Autodesk Inventor part; units mm, degrees
ref_plane "Work Plane1" through (9, 0, 0) normal (1, 0, 0) x (0, 0, -1)
ref_plane "YZ Plane" through (0, 0, 0) normal (1, 0, 0) x (0, 1, 0)
ref_plane "XZ Plane" through (0, 0, 0) normal (0, 1, 0) x (-1, 0, 0)
sketch "Sketch1" plane through (0, 0, 0) normal (1, 0, 0) x (0, 1, 0)
  circle A0 centre (0, 0) radius 1.4
  line L0 (0.5, 1.30767) -> (0.5, -1.30767)
  dimension "d1" = 2.8
  dimension "d2" = 0.5
extrude "Extrusion1" add sketch "Sketch1" along normal blind 8 contours L0 A0 picked at (-0.62029, 0.295862)
sketch "Sketch2" plane through (0, 0, 0) normal (-1, 0, 0) x (0, 0, 1)
  circle A0 centre (0, 0) radius 8.75
  arc A1 (-1.30767, 0.5) -> (1.30767, 0.5) centre (0, 0) ccw
  dimension "d5" = 17.5
extrude "Extrusion2" add sketch "Sketch2" along normal blind 8
sketch "Sketch3" plane through (0, 0, 0) normal (1, 0, 0) x (0, 1, 0)
  circle A0 centre (0, 0) radius 4.25
  line L0 (4, 1.75) -> (8.573214, 1.75)
  line L1 (4, -1.75) -> (8.573214, -1.75)
  line L2 (-10.5, 0) -> (10.5, 0)
  circle A1 centre (0, 0) radius 8.75
  line L3 (0.5, -1.30767) -> (0.5, 1.30767)
  arc A2 (0.5, 1.30767) -> (0.5, -1.30767) centre (0, 0) ccw
  arc A3 (3.820225, 1.86236) -> (4, 1.75) centre (4, 1.95) ccw
  arc A4 (4, -1.75) -> (3.820225, -1.86236) centre (4, -1.95) ccw
  line L4 (-3.515544, 2.589102) -> (-5.802152, 6.549621)
  line L5 (-0.484456, 4.339102) -> (-2.771063, 8.299621)
  arc A5 (-0.484456, 4.339102) -> (-0.297262, 4.239591) centre (-0.31125, 4.439102) ccw
  arc A6 (-3.522963, 2.377232) -> (-3.515544, 2.589102) centre (-3.68875, 2.489102) ccw
  line L6 (-0.484456, -4.339102) -> (-2.771063, -8.299621)
  line L7 (-3.515544, -2.589102) -> (-5.802152, -6.549621)
  arc A7 (-3.515544, -2.589102) -> (-3.522963, -2.377232) centre (-3.68875, -2.489102) ccw
  arc A8 (-0.297262, -4.239591) -> (-0.484456, -4.339102) centre (-0.31125, -4.439102) ccw
  arc A9 (0.5, 1.30767) -> (0.5, -1.30767) centre (0, 0) ccw
  circle A10 centre (0, 0) radius 5
  line L8 (4, 1.75) -> (3.872983, 1.75)
  line L9 (4, -1.75) -> (3.840573, -1.75)
  line L10 (-0.484456, -4.339102) -> (-0.420947, -4.229102)
  line L11 (-3.515544, -2.589102) -> (-3.452036, -2.479102)
  line L12 (-3.515544, 2.589102) -> (-3.452036, 2.479102)
  line L13 (-0.484456, 4.339102) -> (-0.420947, 4.229102)
  point P0 (-3.522963, -2.377232)
  point P1 (-4.25, 0)
  point P2 (-8.75, 0)
  point P3 (-5.802152, -6.549621)
  point P4 (-0.297262, -4.239591)
  point P5 (-2.771063, -8.299621)
  point P6 (8.573214, -1.75)
  point P7 (-0.297262, 4.239591)
  point P8 (-3.522963, 2.377232)
  point P9 (-5.802152, 6.549621)
  point P10 (3.872983, -1.75)
  dimension "d8" = 8.5
  dimension "d9" = 3.5
  dimension "d10" = 4
  dimension "d14" = 360
  dimension "d22" = 10
extrude "Extrusion3" add sketch "Sketch3" along normal blind 8 contours A0 A3 L8 | L9 A4 A0 | A0 A5 L5 A10 L0 A3 | A4 L1 A10 L6 A8 A0 | A10 L5 A1 L0 | L1 A1 L6 A10 | A0 L13 A5 | A8 L10 A0 | L2 A10 L4 A6 A0 | A0 A7 L7 A10 L2 | A10 L2 A1 L4 | L7 A1 L2 A10 | A6 L12 A0 | A0 L11 A7
sketch "Sketch4" plane through (-8, 0, 0) normal (-1, 0, 0) x (0, 0, 1)
  circle A0 centre (0, 0) radius 6.65
  dimension "d19" = 13.3
extrude "Extrusion4" cut sketch "Sketch4" against normal blind 5.5
fillet "Fillet1" radius 3 6 edges at (4, 3.873, 1.75) (4, -0.4209, 4.2291) (4, 3.873, -1.75) (4, -0.4209, -4.2291) (4, -3.452, -2.4791) (4, -3.452, 2.4791)
sketch "Sketch5" plane through (-2.5, 0, 0) normal (-1, 0, 0) x (0, 0, 1)
  circle A0 centre (0, 0) radius 2.5
  dimension "d24" = 5
extrude "Extrusion5" [suppressed]
sketch "Sketch6" plane through (-22, 0, 0) normal (-1, 0, 0) x (0, 0, 1)
  arc A0 (-1.2, 0.5) -> (1.2, 0.5) centre (0, 0) ccw
  circle A1 centre (0, 0) radius 2.5
ref_plane "Work Plane1" through (9, 0, 0) normal (1, 0, 0) x (0, 0, -1)
sketch "Sketch7" plane through (9, 0, 0) normal (1, 0, 0) x (0, 0, -1)
  arc A0 (-1.30767, 0.5) -> (1.30767, 0.5) centre (0, 0) ccw
  line L0 (1.30767, 0.5) -> (-1.30767, 0.5)
  circle A1 centre (0, 0) radius 1.6
  line L1 (-1.438749, 0.7) -> (1.438749, 0.7)
  dimension "d28" = 3.2
  dimension "d30" = 0.5
  dimension "d31" = 0.7
sketch "Sketch8" plane through (8, 0, 0) normal (1, 0, 0) x (0, 0, -1)
  arc A0 (-1.30767, 0.5) -> (1.30767, 0.5) centre (0, 0) ccw
  line L0 (1.30767, 0.5) -> (-1.30767, 0.5)
sketch "Sketch7 outline for Loft1" plane through (9, 0, 0) normal (1, 0, 0) x (0, 0, -1)
  line L0 (1.438749, 0.7) -> (-1.438749, 0.7)
  arc A0 (-1.438749, 0.7) -> (1.438749, 0.7) centre (0, 0) ccw
loft "Loft1" add profiles "Sketch7 outline for Loft1" section 1 edges at (8, -1.4, 0) (8, 0.5, 0)
sketch "Sketch9" plane through (-2.5, 0, 0) normal (-1, 0, 0) x (0, 0, 1)
  circle A0 centre (0, 0) radius 3.15
  dimension "d36" = 6.3
extrude "Extrusion6" cut sketch "Sketch9" against normal blind 0.4
properties part number "front wheel mount"
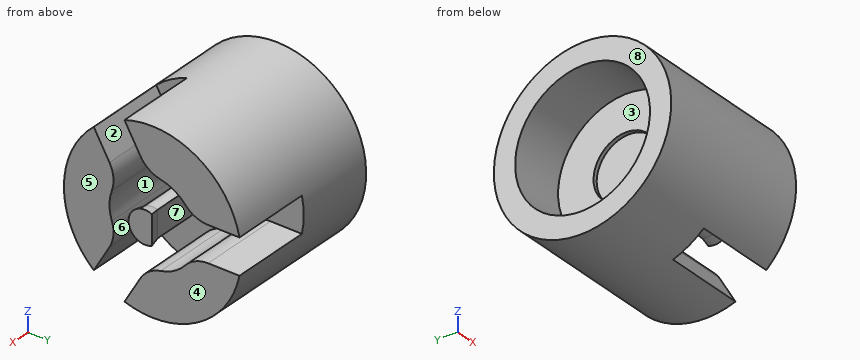
Verification items for the finished model (mm, model axes). Face numbers are marked on the shaded views. A direction names the side the tool comes from. Coordinates: 2 decimals unless noted, no trailing zeros. Write each loop counter-clockwise with the first axis right and the second up, starting at its lowest first coordinate (ties: lowest second). Pieces come first, ordered by that corner, then holes. Notation, with made-up numbers: (40.5, -9.75) -> (99.5, -9.75) arc R25 ccw to (99.5, 24.25) -> close; hole circle Ø9 at (3.25, -18.75). An arc over 180 degrees is marked (long way). One line per item, written item: value. Start each with the question number.
Q1. Cross-section at C-C on x = -5. Enter the section's corners in (y, z), and give its area (3 significant figures).
Q2. Cross-section at A-A on x = 6.25. Enter the section's corners in (y, z) (3 decimals).
Q3. Cross-section at D-D on z = -7. Enter the section's corners in (x, y).
Q4. Mould release check, pull along Y, two halves, no side actions. Record for the marked faces 6, 7 and 8: pulls with the +Y half, pulls with the -Y half, needs draft (parallel to the pull), parting line crosses it, or undercut.
Q5. Cross-section at B-B on y = -4.5. Enter the section's corners in (x, z), and give its area (3 significant figures).
Q6. Go/stop test with flat-tipped pins: P1, Ø4, axis at y = -0.5, z = -3, coming from the -X side; P2, Ø2, axis at x = 0, y = -4, coming from the -Z side; P3, Ø8, axis at x = 0, y = 5, coming from the -Z side. Record where each tip stops, or that it passes through.
Q7. Thickness scan on L1, parallel to Y at x = -5.4, z = 0; L2, parallel to Y at x = -2.4, z = 0; L3, parallel to Z at x = 1, y = -1.75. Record the ranges inside material, lowest first. Write a range as from..to.
Q8. Access from +Z, -Z, +X, -X, +Y, -Y to the whole of each face (thin tool, end or side, straight path). Record for the marked faces 1, 2, 3, 4 and 5.
Checked values:
1. outline: circle Ø17.5 at (0, 0); hole circle Ø13.3 at (0, 0)
1. area: 102 mm²
2. outline: (-5.802, -6.55) -> (-4.254, -3.868) arc R3 ccw to (-4.017, -1.388) arc R4.25 cw to (-4.017, 1.388) arc R3 ccw to (-4.254, 3.868) -> (-5.802, 6.55) arc R8.75 ccw to start; (-2.771, -8.3) arc R8.75 ccw to (8.573, -1.75) -> (5.477, -1.75) arc R3 ccw to (3.211, -2.784) arc R4.25 cw to (0.806, -4.173) arc R3 ccw to (-1.223, -5.618) -> close; (-2.771, 8.3) -> (-1.223, 5.618) arc R3 ccw to (0.806, 4.173) arc R4.25 cw to (3.211, 2.784) arc R3 ccw to (5.477, 1.75) -> (8.573, 1.75) arc R8.75 ccw to start; (0.5, -1.308) -> (0.5, 1.308) arc R1.4 ccw (long way) to start
3. outline: (-8, -5.25) -> (0, -5.25) -> (0, -2.02) -> (8, -2.02) -> (8, 5.25) -> (-8, 5.25) -> close
4. face 6: undercut
4. face 7: pulls with the +Y half
4. face 8: needs draft
5. outline: (-8, -7.5) -> (0, -7.5) -> (0, -4.29) -> (8, -4.29) -> (8, 4.29) -> (0, 4.29) -> (0, 7.5) -> (-8, 7.5) -> (-8, 4.9) -> (-2.5, 4.9) -> (-2.5, -4.9) -> (-8, -4.9) -> close
5. area: 135 mm²
6. P1: stops at x = -2.5
6. P2: stops at z = -8.22
6. P3: stops at z = -8.69
7. L1: y = -8.75..-6.65, 6.65..8.75
7. L2: y = -8.75..-3.15, 3.15..8.75
7. L3: z = -8.57..-6.53, 6.53..8.57
8. face 1: +X
8. face 2: +Z, +X
8. face 3: -X
8. face 4: -Z, +X, +Y, -Y
8. face 5: +Z, -Z, +X, -Y
